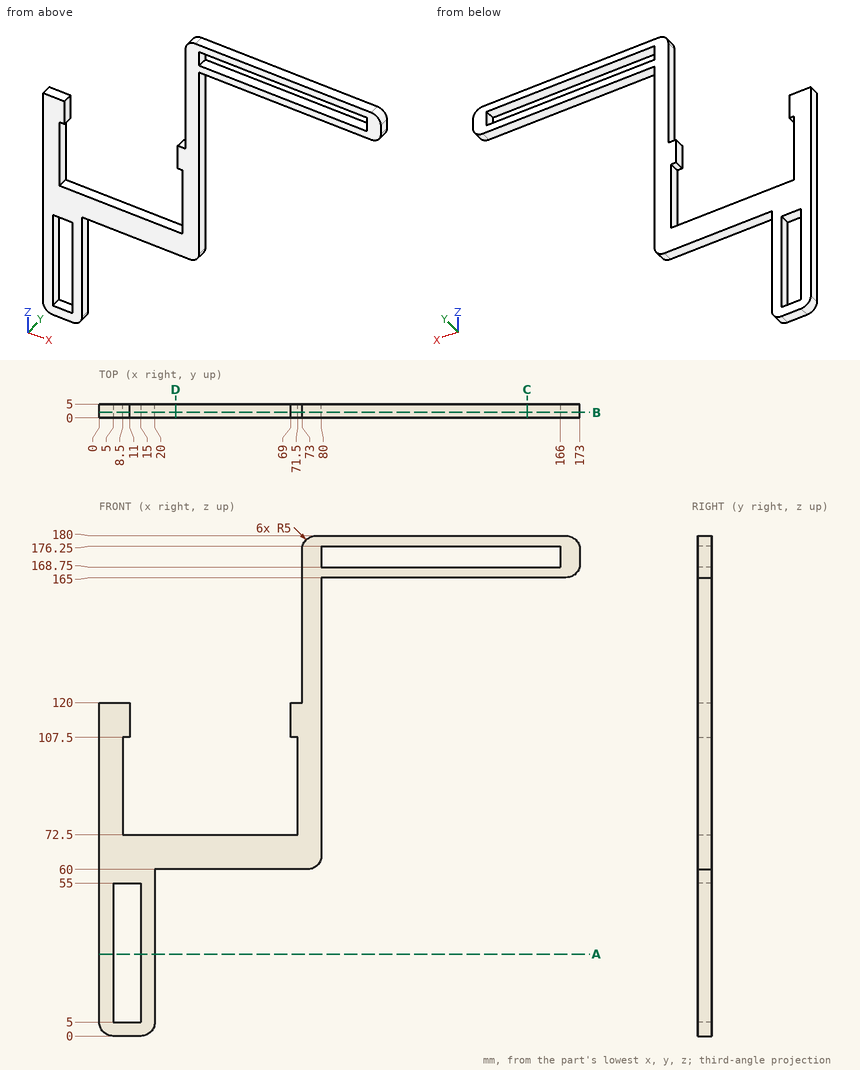
Check sheet for the drawn part. Datum: minimum x, y, z corner. Units: mm. Round coordinates to 2 decimals unless told otherwise and drop trailing zeros. Write each loop counter-clockwise with the first axis right and the second up, starting at its lowest first coordinate (ties: lowest second). Pieces come first, ordered by that corner, then holes. Notation, with made-up numbers: (-15.75, 21.25) -> (17.25, 21.25) arc R13 ccw to (17.25, 31.25) -> close; hole circle Ø9 at (78, 42). An arc over 180 degrees is marked (long way). Write each question's results on one line, items separated by ' | '.
Q1. Sectioned sample at D-D, the plane x = 27.5. Record the boundary of the cut face in (y, z), and give its area (3 significant figures).
Derived:
outline: (0, 60) -> (5, 60) -> (5, 72.5) -> (0, 72.5) -> close | area: 62.5 mm²
Q2. Sectioned sample at B-B, the plane y = 2. Give the number of separate pieces and of enclosed holes in the cut face, and give its area (3 significant figures).
Derived:
separate pieces: 1 | enclosed holes: 2 | area: 3,710 mm²
Q3. Sectioned sample at C-C, the plane x = 154. Record the boundary of the cut face in (y, z).
Derived:
outline: (0, 165) -> (5, 165) -> (5, 168.75) -> (0, 168.75) -> close; (0, 176.25) -> (5, 176.25) -> (5, 180) -> (0, 180) -> close
Q4. Thickness scan on probe 1 along X at (y, z) = (0.8, 82); probe 2 along Z at (x, y) = (83.5, 2.45); probe 3 along X at (y, z) = (3.7, 43). Record the ranges inside material, lowest first.
Derived:
probe 1: x = 0 to 8.5, 71.5 to 80 | probe 2: z = 165 to 168.75, 176.25 to 180 | probe 3: x = 0 to 5, 15 to 20
Q5. Sectioned sample at A-A, the plane z = 29.5. Record the boundary of the cut face in (x, y), and give its area (3 significant figures).
Derived:
outline: (0, 0) -> (5, 0) -> (5, 5) -> (0, 5) -> close; (15, 0) -> (20, 0) -> (20, 5) -> (15, 5) -> close | area: 50.0 mm²
Q6. Go/stop test with flat-tipped pins: pin 1 Ø2.5 at (x, y) = (39.5, 3) entering from -Z; pin 2 Ø1.5 at (y, z) = (4.5, 123) entering from +X; pin 3 Ø3 at (y, z) = (3, 141.5) entering from -X. Record where each tip stops, or that it passes through.
Derived:
pin 1: stops at z = 60 | pin 2: stops at x = 80 | pin 3: stops at x = 73
